Here's the drawing with two shaded views (mm, measured from the low corner). I have some questions. A direction names the side the tool comes from. Round coordinates to 2 decimals unless told otherwise and drop trailing zeros. Loops run counter-clockwise (first coordinate to the right, second up) from the corner with the lowest first, then second, coordinate; pieces in that order, holes last. Notation, with made-up numbers: (59.25, -25) -> (116.25, -25) arc R23 ccw to (116.25, -16) -> close; hole circle Ø5 at (9, -15.75). An arc over 180 degrees is marked (long way). Write each question's results on one line, items separated by ' | '. Start each with the question number.
1) Imagine slicing it at D-D, the plane z = 6.75. List the corners of the cut face in (x, y) for me, plus the area to 3 significant figures.
2) Imagine slicing it at B-B, the plane z = 4. List the corners of the cut face in (x, y) for me.
3) If I drill on probe 1 along Y at (x, z) = (3, 6); probe 2 along Y at (x, z) = (7.25, 7); probe 3 along X at (y, z) = (6.25, 4), over which ranges is the centre line in solid material (lowest first)?
4) Imagine slicing it at A-A, the plane x = 6. List the corners of the cut face in (y, z) for me, plus the area to 3 significant figures.
5) Which directions (+Z, -Z, +X, -X, +Y, -Y) give clear straight access to the entire face, cutting with the end or side of a thin tool? Please do the marked faces 1 and 2.
6) Imagine slicing it at C-C, the plane y = 5.25. List the corners of the cut face in (x, z) for me.
7) For P1, Ø4, axis at y = 5, z = 2.5, coming from the +X side, with a flat end and sliding along its axis, tell me the tip position at first contact or that it passes through.
8) We'd pull the mould along X, two halves only. Please class the marked faces 3, 4 and 5: pulls with the +X half, pulls with the -X half, needs draft (parallel to the pull), parting line crosses it, or undercut.
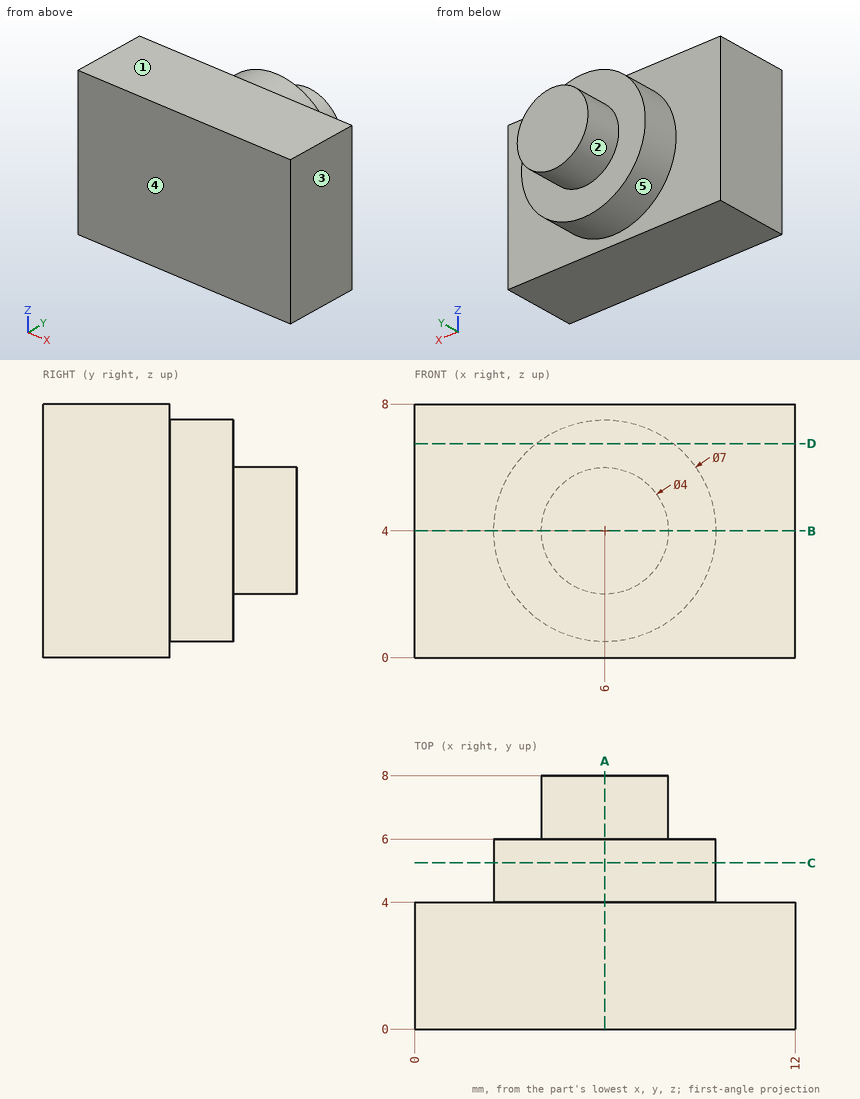
Checked values:
1) outline: (0, 0) -> (12, 0) -> (12, 4) -> (8.17, 4) -> (8.17, 6) -> (3.83, 6) -> (3.83, 4) -> (0, 4) -> close | area: 56.7 mm^2
2) outline: (0, 0) -> (12, 0) -> (12, 4) -> (9.5, 4) -> (9.5, 6) -> (8, 6) -> (8, 8) -> (4, 8) -> (4, 6) -> (2.5, 6) -> (2.5, 4) -> (0, 4) -> close
3) probe 1: 0 to 4 | probe 2: 0 to 6 | probe 3: 4 to 8
4) outline: (0, 0) -> (4, 0) -> (4, 0.5) -> (6, 0.5) -> (6, 2) -> (8, 2) -> (8, 6) -> (6, 6) -> (6, 7.5) -> (4, 7.5) -> (4, 8) -> (0, 8) -> close | area: 54.0 mm^2
5) face 1: +Z, +X, -X, +Y, -Y | face 2: +Y
6) outline: circle Ø7 at (6, 4)
7) P1: x = 12
8) face 3: pulls with the +X half | face 4: needs draft | face 5: parting line crosses it
